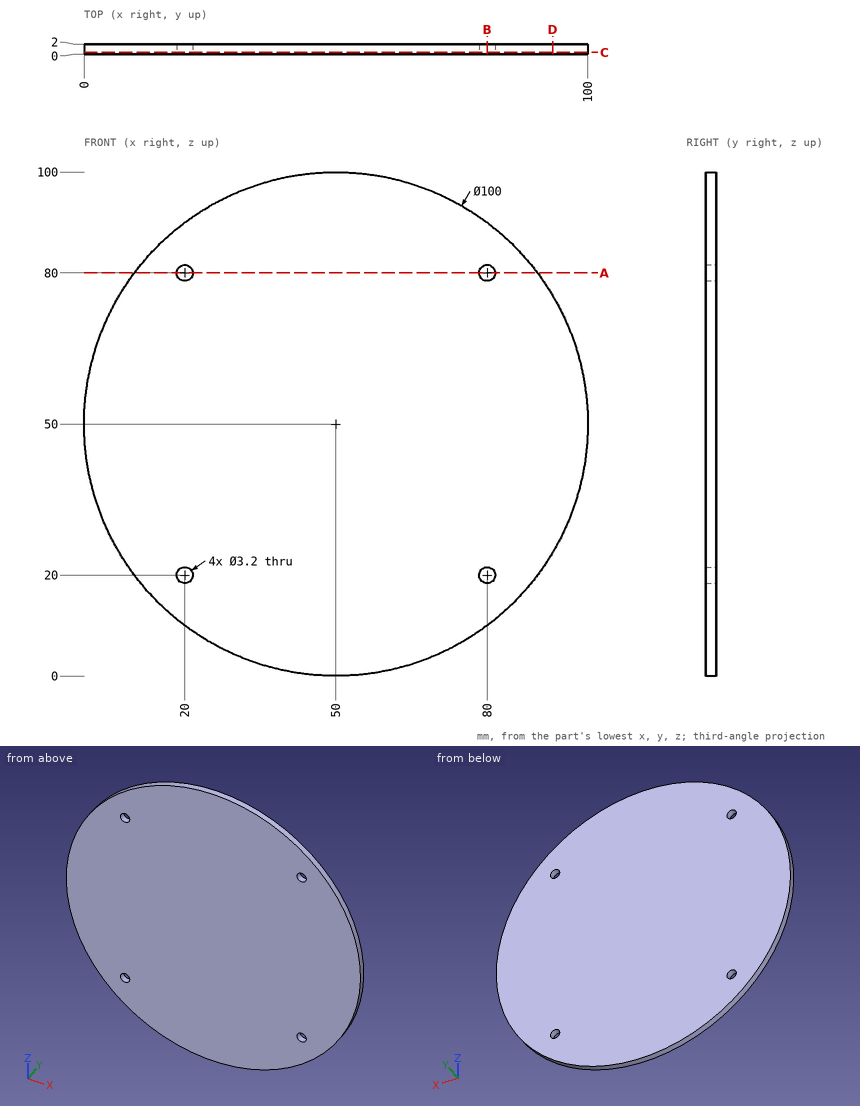
Design review of the part shown in the three views and the two pictorial views. Dimensions are in mm from the part's minimum x, y and z. Give positions to 0.01 mm unless a question says otherwise; leave off trailing zeros. Loops run counter-clockwise (first coordinate to the right, second up) from the corner with the lowest first, then second, coordinate; pieces in that order, holes last. Notation, with made-up numbers: (61, -33.75) -> (111, -33.75) arc R15 cw to (111, -13.75) -> close; hole circle Ø8 at (-38.5, 80). An arc over 180 degrees is marked (long way). Answer as a JSON object with one key per item and string values. Group by question number.
Q1. Take a section at D-D (x = 93). Write out the cut boundary in (y, z), plus the area to 3 significant figures.
Q2. Take a section at C-C (y = 0.35). Write out the cut boundary in (x, z).
Q3. Take a section at B-B (x = 80). Write out the cut boundary in (y, z), plus the area to 3 significant figures.
Q4. Insertion check: pin 1 (12 mm diameter, centred on x = 47, z = 11, fed in from -Y). The pin has a flat end and moves straight along its axis. Give the tip position at first contact, or say it passes through.
Q5. Take a section at A-A (z = 80). Write out the cut boundary in (x, y), plus the area to 3 significant figures.
Q6. Wall thickness on line 1 along Z through (x, y) = (80, 0.15); line 2 along X through (y, z) = (0.85, 79.5): over which ranges is each line inside the solid? List them lowest first.
Answer below:
{
 "1": {"outline": "(0, 24.49) -> (2, 24.49) -> (2, 75.51) -> (0, 75.51) -> close", "area": "102 mm2"},
 "2": {"outline": "circle Ø100 at (50, 50); hole circle Ø3.2 at (20, 20); hole circle Ø3.2 at (20, 80); hole circle Ø3.2 at (80, 20); hole circle Ø3.2 at (80, 80)"},
 "3": {"outline": "(0, 10) -> (2, 10) -> (2, 18.4) -> (0, 18.4) -> close; (0, 21.6) -> (2, 21.6) -> (2, 78.4) -> (0, 78.4) -> close; (0, 81.6) -> (2, 81.6) -> (2, 90) -> (0, 90) -> close", "area": "147 mm2"},
 "4": {"pin 1": "stops at y = 0"},
 "5": {"outline": "(10, 0) -> (18.4, 0) -> (18.4, 2) -> (10, 2) -> close; (21.6, 0) -> (78.4, 0) -> (78.4, 2) -> (21.6, 2) -> close; (81.6, 0) -> (90, 0) -> (90, 2) -> (81.6, 2) -> close", "area": "147 mm2"},
 "6": {"line 1": "z = 10 to 18.4, 21.6 to 78.4, 81.6 to 90", "line 2": "x = 9.63 to 18.48, 21.52 to 78.48, 81.52 to 90.37"}
}
